```python
from build123d import *

# Parameters (mm, degrees)
F1_DEPTH = 76.2
F3_DEPTH = 63.5
F4_R     = 14.889155
F5_DEPTH = 203.2


with BuildPart() as f1:
    # F0 (on Front) → F1 (new body)
    with BuildSketch(Plane.XZ):
        Polygon((-24.165607, 74.374091), (-78.201547, 0), (-24.165607, -74.374091), (63.266381, -45.965716), (63.266381, 45.965716), align=None)
    extrude(amount=F1_DEPTH)

    # F2 (on face) → F3 (cut)
    with BuildSketch(Plane(origin=(0, 0, 0), x_dir=(-1, 0, 0), z_dir=(0, 1, 0))):
        Polygon((-23.337874, 45.790973), (-50.761603, -8.045448), (-8.034522, -50.763333), (45.795995, -23.328017), (36.338004, 36.345826), align=None)
    extrude(amount=-F3_DEPTH, mode=Mode.SUBTRACT)

    # F4 (on face) → F5 (join)
    with BuildSketch(Plane(origin=(0, -63.5, 0), x_dir=(-1, 0, 0), z_dir=(0, 1, 0))):
        with Locations((-4.347364, 0)):
            Circle(F4_R)
    extrude(amount=F5_DEPTH)


solid = f1.part
```
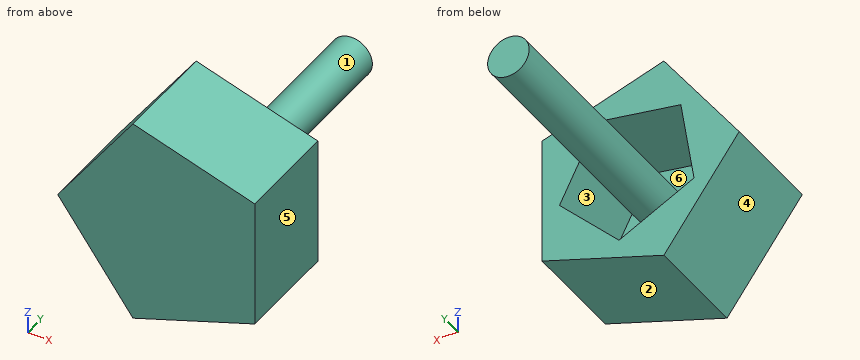
Read the model definition and answer for the solid it produces. Units are mm, in the model's axes. Face numbers are marked on the shaded views. A direction names the side the tool comes from. Give positions to 0.01 mm unless a question says otherwise; leave off trailing zeros. Write each loop counter-clockwise with the first axis right and the second up, starting at its lowest first coordinate (ties: lowest second). Pieces come first, ordered by that corner, then holes. Notation, with made-up numbers: (-29, 77.25) -> (-13, 77.25) arc R19 cw to (-13, 105.25) -> close; hole circle Ø4 at (-38.75, 26). An arc over 180 degrees is marked (long way). Answer in a Markdown table with one row per item.
1) Section A-A on x = 27 is taken. Give the vertices of the cut face in (y, z).
Results list:
| item | result |
|---|---|
| outline | (-76.2, -57.75) -> (0, -57.75) -> (0, -31.8) -> (-63.5, -31.8) -> (-63.5, 38.6) -> (0, 38.6) -> (0, 57.75) -> (-76.2, 57.75) -> close |
2) Straight lines are drawn through the part: line 1 (Z direction, x = -7.5, y = -36); line 2 (Z direction, x = 2.5, y = -8); line 3 (Y direction, x = -35, z = -23). For each, find the intervals that lie inside material, in ascending order. Write a range as [from, to].
Results list:
| item | result |
|---|---|
| line 1 | [-68.96, -42.85], [-9.02, 9.02], [40.91, 68.96] |
| line 2 | [-65.71, -47.94], [-14.77, 14.77], [42.49, 65.71] |
| line 3 | [-76.2, -63.5] |
3) Section D-D on z = 3 is taken. Give the vertices of the cut face in (x, y).
Results list:
| item | result |
|---|---|
| outline | (-76.02, -76.2) -> (63.27, -76.2) -> (63.27, 0) -> (45.14, 0) -> (45.14, -63.5) -> (18.93, -63.5) -> (18.93, 139.7) -> (-10.24, 139.7) -> (-10.24, -63.5) -> (-41.62, -63.5) -> (-41.62, 0) -> (-76.02, 0) -> close |
4) Determine the mould class of the marked faces 3, 4, 5 and 6 for opening direction Z: released by +Z, released by -Z, zero draft, split by the parting line, or undercut.
Results list:
| item | result |
|---|---|
| face 3 | undercut |
| face 4 | released by -Z |
| face 5 | zero draft |
| face 6 | undercut |
5) A tool of negligible diameter and unlimited length cuts with its end or side. For the marked faces 1 and 2, from which of +Z, -Z, +X, -X, +Y, -Y can it reach the whole face along a straight path? Write none if from no direction.
Results list:
| item | result |
|---|---|
| face 1 | +Y |
| face 2 | -Z, +X, +Y, -Y |
6) Each of these flat-tipped pins is pushed along its axis until it touches: pin 1 Ø12 at (y, z) = (-24.5, -39) entering from -X; pin 2 Ø8 at (x, y) = (-6, -0.5) entering from -Z; pin 3 Ø12 at (x, y) = (2.5, -15) entering from -Z. Where does it stop, or does it pass through?
Results list:
| item | result |
|---|---|
| pin 1 | x = -54.23 |
| pin 2 | z = -69.77 |
| pin 3 | z = -67.66 |
7) Section C-C on y = 85 is taken. Give the vertices of the cut face in (x, z).
Results list:
| item | result |
|---|---|
| outline | circle Ø29.78 at (4.35, 0) |
8) Section B-B on z = -38 is taken. Give the vertices of the cut face in (x, y), plus the area to 3 significant figures.
Results list:
| item | result |
|---|---|
| outline | (-50.59, -76.2) -> (63.27, -76.2) -> (63.27, 0) -> (20.8, 0) -> (20.8, -63.5) -> (-17.01, -63.5) -> (-17.01, 0) -> (-50.59, 0) -> close |
| area | 6,280 mm^2 |
